```python
from build123d import *

# Parameters (mm, degrees)
SKETCH6_W               = 120
SKETCH6_H               = 27
BASE_FLANGE2_DEPTH      = 1
EDGE_FLANGE1_DEPTH      = 27
EDGE_FLANGE1_BEND_DEPTH = 27
EDGE_FLANGE2_DEPTH      = 20
EDGE_FLANGE3_DEPTH      = 20
CUT_EXTRUDE1_REACH      = 136.321
SKETCH26_R              = 1.4
CUT_EXTRUDE2_REACH      = 75.526
SKETCH27_R              = 1.4
BREAK_CORNER1_START     = -61.7366
BREAK_CORNER1_DEPTH     = 123.4732
CUT_EXTRUDE3_REACH      = 83.289


# Read off the part's stored shape, not the designer's step: Break-Corner1
# Sheet-metal steps are written as plain solids
with BuildPart() as part:
    # Sketch6 → Base-Flange2 (new body)
    with BuildSketch(Plane(origin=(0, 0, 0), x_dir=(1, 0, 0), z_dir=(0, 1, 0))):
        Rectangle(SKETCH6_W, SKETCH6_H)
    extrude(amount=-BASE_FLANGE2_DEPTH)

    # Edge-Flange1 section (across the edge) → Edge-Flange1 (add)
    with BuildSketch(Plane(origin=(-60.7366, 0, -13.5), x_dir=(1, 0, 0), z_dir=(0, 0, 1))):
        with BuildLine():
            Line((-1, 0.7366), (-1, 47))
            Line((-1, 47), (0, 47))
            Line((0, 47), (0, 0.7366))
            ThreePointArc((0, 0.7366), (0.215745145, 0.215745145), (0.7366, 0))
            Line((0.7366, 0), (0.7366, -1))
            ThreePointArc((0.7366, -1), (-0.491361636, -0.491361636), (-1, 0.7366))
        make_face()
    extrude(amount=EDGE_FLANGE1_DEPTH)

    # Edge-Flange1 section 2 (across the edge) → Edge-Flange1 bend (add)
    with BuildSketch(Plane(origin=(60.7366, 0, 13.5), x_dir=(-1, 0, 0), z_dir=(0, 0, -1))):
        with BuildLine():
            Line((-1, 0.7366), (-1, 47))
            Line((-1, 47), (0, 47))
            Line((0, 47), (0, 0.7366))
            ThreePointArc((0, 0.7366), (0.215745145, 0.215745145), (0.7366, 0))
            Line((0.7366, 0), (0.7366, -1))
            ThreePointArc((0.7366, -1), (-0.491361636, -0.491361636), (-1, 0.7366))
        make_face()
    extrude(amount=EDGE_FLANGE1_BEND_DEPTH)

    # Edge-Flange2 section (across the edge) → Edge-Flange2 (add)
    with BuildSketch(Plane(origin=(-36.7366, 0, 14.2366), x_dir=(0, 0, -1), z_dir=(1, 0, 0))):
        with BuildLine():
            Line((-1, 0.7366), (-1, 29))
            Line((-1, 29), (0, 29))
            Line((0, 29), (0, 0.7366))
            ThreePointArc((0, 0.7366), (0.215745145, 0.215745145), (0.7366, 0))
            Line((0.7366, 0), (0.7366, -1))
            ThreePointArc((0.7366, -1), (-0.491361636, -0.491361636), (-1, 0.7366))
        make_face()
    extrude(amount=EDGE_FLANGE2_DEPTH)

    # Edge-Flange3 section (across the edge) → Edge-Flange3 (add)
    with BuildSketch(Plane(origin=(-16.7366, 29.7366, 15.2366), x_dir=(0, -1, 0), z_dir=(-1, 0, 0))):
        with BuildLine():
            Line((-1, 0.7366), (-1, 9))
            Line((-1, 9), (0, 9))
            Line((0, 9), (0, 0.7366))
            ThreePointArc((0, 0.7366), (0.215745145, 0.215745145), (0.7366, 0))
            Line((0.7366, 0), (0.7366, -1))
            ThreePointArc((0.7366, -1), (-0.491361636, -0.491361636), (-1, 0.7366))
        make_face()
    extrude(amount=EDGE_FLANGE3_DEPTH)

    # Sketch26 → Cut-Extrude1 (cut, up to next)
    with BuildSketch(Plane(origin=(61.7366, 0, 0), x_dir=(0, 0, -1), z_dir=(1, 0, 0)), mode=Mode.PRIVATE) as cut_extrude1_sk1:
        with Locations(Location((-7.5, 42.419132502, 0), (0, 0, 90))):
            Circle(SKETCH26_R)
    cut_extrude1_tool1 = extrude(cut_extrude1_sk1.sketch, amount=-CUT_EXTRUDE1_REACH, mode=Mode.PRIVATE) & part.part
    # Sketch26 → Cut-Extrude1 (cut, up to next)
    with BuildSketch(Plane(origin=(61.7366, 0, 0), x_dir=(0, 0, -1), z_dir=(1, 0, 0)), mode=Mode.PRIVATE) as cut_extrude1_sk2:
        with Locations(Location((0, 42.419132502, 0), (0, 0, 90))):
            Circle(SKETCH26_R)
    cut_extrude1_tool2 = extrude(cut_extrude1_sk2.sketch, amount=-CUT_EXTRUDE1_REACH, mode=Mode.PRIVATE) & part.part
    # Sketch26 → Cut-Extrude1 (cut, up to next)
    with BuildSketch(Plane(origin=(61.7366, 0, 0), x_dir=(0, 0, -1), z_dir=(1, 0, 0)), mode=Mode.PRIVATE) as cut_extrude1_sk3:
        with Locations(Location((7.5, 42.419132502, 0), (0, 0, 90))):
            Circle(SKETCH26_R)
    cut_extrude1_tool3 = extrude(cut_extrude1_sk3.sketch, amount=-CUT_EXTRUDE1_REACH, mode=Mode.PRIVATE) & part.part
    cut_extrude1_1 = cut_extrude1_tool1.solids().sort_by_distance((61.7366, 42.419133, 7.5))[0]
    add(cut_extrude1_1, mode=Mode.SUBTRACT)
    cut_extrude1_2 = cut_extrude1_tool2.solids().sort_by_distance((61.7366, 42.419133, 0))[0]
    add(cut_extrude1_2, mode=Mode.SUBTRACT)
    cut_extrude1_3 = cut_extrude1_tool3.solids().sort_by_distance((61.7366, 42.419133, -7.5))[0]
    add(cut_extrude1_3, mode=Mode.SUBTRACT)
    cut_extrude1 = cut_extrude1_1 + cut_extrude1_2 + cut_extrude1_3  # Cut-Extrude1 as one shape, for the pattern or mirror that repeats it

    # Mirror1: Cut-Extrude1 across plane
    add(cut_extrude1.mirror(Plane(origin=(0, 0, 0), x_dir=(0, 0, 1), z_dir=(1, 0, 0))), mode=Mode.SUBTRACT)

    # Sketch27 → Cut-Extrude2 (cut, up to next)
    with BuildSketch(Plane(origin=(0, 30.7366, 0), x_dir=(1, 0, 0), z_dir=(0, 1, 0)), mode=Mode.PRIVATE) as cut_extrude2_sk1:
        with Locations(Location((-31.7366, -20.2366, 0), (0, 0, 270))):
            Circle(SKETCH27_R)
    cut_extrude2_tool1 = extrude(cut_extrude2_sk1.sketch, amount=-CUT_EXTRUDE2_REACH, mode=Mode.PRIVATE) & part.part
    # Sketch27 → Cut-Extrude2 (cut, up to next)
    with BuildSketch(Plane(origin=(0, 30.7366, 0), x_dir=(1, 0, 0), z_dir=(0, 1, 0)), mode=Mode.PRIVATE) as cut_extrude2_sk2:
        with Locations(Location((-21.7366, -20.2366, 0), (0, 0, 270))):
            Circle(SKETCH27_R)
    cut_extrude2_tool2 = extrude(cut_extrude2_sk2.sketch, amount=-CUT_EXTRUDE2_REACH, mode=Mode.PRIVATE) & part.part
    add(cut_extrude2_tool1.solids().sort_by_distance((-31.7366, 30.7366, 20.2366))[0], mode=Mode.SUBTRACT)
    add(cut_extrude2_tool2.solids().sort_by_distance((-21.7366, 30.7366, 20.2366))[0], mode=Mode.SUBTRACT)

    # Break-Corner1 outline → Break-Corner1 (cut)
    with BuildSketch(Plane.YZ.offset(BREAK_CORNER1_START)):
        Polygon((47, -13.5), (47, -9.5), (43, -13.5), align=None)
        Polygon((43, 13.5), (47, 9.5), (47, 13.5), align=None)
    extrude(amount=BREAK_CORNER1_DEPTH, mode=Mode.SUBTRACT)

    # Sketch29 → Cut-Extrude3 (cut, up to next)
    with BuildSketch(Plane(origin=(0, 0, 0), x_dir=(1, 0, 0), z_dir=(0, 1, 0)), mode=Mode.PRIVATE) as cut_extrude3_sk1:
        with BuildLine():
            Line((-34.494615607, 12.065428481), (-34.361517182, 11.934571519))
            ThreePointArc((-34.361517182, 11.934571519), (-32.749919682, 10.872519994), (-30.856132789, 10.5))
            Line((-30.856132789, 10.5), (30.858555604, 10.5))
            ThreePointArc((30.858555604, 10.5), (32.791568542, 10.888767954), (34.423984085, 11.994615607))
            Line((34.423984085, 11.994615607), (34.434571519, 12.005384393))
            ThreePointArc((34.434571519, 12.005384393), (36.066987062, 13.111232046), (38, 13.5))
            Line((38, 13.5), (-38, 13.5))
            ThreePointArc((-38, 13.5), (-36.106213107, 13.127480006), (-34.494615607, 12.065428481))
        make_face()
    cut_extrude3_tool1 = extrude(cut_extrude3_sk1.sketch, amount=-CUT_EXTRUDE3_REACH, mode=Mode.PRIVATE) & part.part
    add(cut_extrude3_tool1.solids().sort_by_distance((0.000586, 0, -12.034279))[0], mode=Mode.SUBTRACT)


solid = part.part
```
Model file for the job. Use its own axes, mm. A direction names the side the tool comes from. Give positions to 0.01 mm unless a question says otherwise; leave off trailing zeros. Write each loop counter-clockwise with the first axis right and the second up, starting at its lowest first coordinate (ties: lowest second). Pieces come first, ordered by that corner, then holes. Notation, with made-up numbers: M 9.25,89.25 L 15.25,89.25 A21 ccw 15.25,128.25 Z; hole C 9,9 d1. An arc over 180 degrees is marked long. Use a Markdown table: item, result.
1) Pull direction Y, two halves, no side cores. Call faces 1 (the cylindrical face through (-30.79, 30.244, 19.205)), 2 (the cylindrical face through (-61.24, 41.02, 7.56)), 3 (the flat face through (61.2, 45, -11.5)): +Y half, -Y half, draft (parallel to the pull), parting line (faces both ways), or undercut.
Responses:
| item | result |
|---|---|
| face 1 | draft |
| face 2 | undercut |
| face 3 | +Y half |
2) Drill centre lines: line 1 (X direction, y = 26.5, z = -2); line 2 (Y direction, x = -44.5, z = -3.5); line 3 (Z direction, x = -17.5, y = 7.5). Where is each one in solid material? Low to high. Write a range as from..to.
Responses:
| item | result |
|---|---|
| line 1 | x = -61.74..-60.74, 60.74..61.74 |
| line 2 | y = -1..0 |
| line 3 | z = 14.24..15.24 |
3) Cut at C-C (y = 6). List the corners of the cut face in (x, z), and give its area (3 significant figures).
Responses:
| item | result |
|---|---|
| outline | M -61.74,-13.5 L -60.74,-13.5 L -60.74,13.5 L -61.74,13.5 Z; M -36.74,14.24 L -16.74,14.24 L -16.74,15.24 L -36.74,15.24 Z; M 60.74,-13.5 L 61.74,-13.5 L 61.74,13.5 L 60.74,13.5 Z |
| area | 74.0 mm2 |
4) Cut at A-A (z = 0). List the corners of the cut face in (x, y).
Responses:
| item | result |
|---|---|
| outline | M -61.74,0.74 A1.74 ccw -60,-1 L 60,-1 A1.74 ccw 61.74,0.74 L 61.74,41.02 L 60.74,41.02 L 60.74,0.74 A0.74 cw 60,0 L -60,0 A0.74 cw -60.74,0.74 L -60.74,41.02 L -61.74,41.02 Z; M -61.74,43.82 L -60.74,43.82 L -60.74,47 L -61.74,47 Z; M 60.74,43.82 L 61.74,43.82 L 61.74,47 L 60.74,47 Z |
5) Cut at B-B (y = 35). List the corners of the cut face in (x, z), and give its area (3 significant figures).
Responses:
| item | result |
|---|---|
| outline | M -61.74,-13.5 L -60.74,-13.5 L -60.74,13.5 L -61.74,13.5 Z; M 60.74,-13.5 L 61.74,-13.5 L 61.74,13.5 L 60.74,13.5 Z |
| area | 54.0 mm2 |
6) Tool access for faces 4 (the flat face through (-27, 15, 15.237)), 5 (the flat face through (60.737, 24, 0)), 6 (the flat face through (61.2, 45, 11.5)), 7 (the flat face through (-61, 11, 13.5)), 8 (the cylindrical face through (61.24, 41.02, 7.56)): list every direction of +Z, -Z, +X, -X, +Y, -Y with a clear straight run to the whole face (end or side of a thin tool).
Responses:
| item | result |
|---|---|
| face 4 | +Z, +X, -X, -Y |
| face 5 | +Z, -Z, +Y |
| face 6 | +Z, +X, -X, +Y |
| face 7 | +Z, -X, +Y, -Y |
| face 8 | +X, -X |
7) Pin check, flat tips, straight feed: pin 1 (4.5 mm diameter, centred on x = -21.74, z = 20.24, fed in from -Y); pin 2 (10 mm diameter, centred on x = -40.5, y = 12.5, fed in from +Z); pin 3 (2.5 mm diameter, centred on y = 42.42, z = 0, fed in from -X); pin 4 (2.5 mm diameter, centred on x = -25.5, z = 19.5, fed in from +Y). Stop position of each tip, or through.
Responses:
| item | result |
|---|---|
| pin 1 | stops at y = 29.74 |
| pin 2 | stops at z = 15.24 |
| pin 3 | passes through |
| pin 4 | stops at y = 30.74 |
